For this review, take the finished solid that the model builds, in its own axes (mm). A direction names the side the tool comes from. Round coordinates to 2 decimals unless told otherwise and drop trailing zeros. Write each loop counter-clockwise with the first axis right and the second up, starting at its lowest first coordinate (ties: lowest second). Pieces come first, ordered by that corner, then holes. Notation, with made-up numbers: (64, 67.25) - (81, 67.25) arc R26 cw to (81, 97.25) - close; hole circle Ø9 at (20.25, 59.5). An arc over 180 degrees is marked (long way). One line per item, written item: value. Start each with the question number.
Q1. Mouldability with a two-part tool opening along Y and no side actions: class faces 3 (the face through (-0.524, 1.61, 1.663)), 4 (the face through (0, 6, 0)), 5 (the face through (-0.871, 3.481, 2.766)), 6 (the face through (-0.2, -0.3, 0.7)) as +Y half, -Y half, draft (parallel to the pull), parting line (faces both ways), or undercut.
Q2. Add section B-B on y = 4. Write out the cut boundary in (x, z).
Q3. Add section A-A on y = 0.25. Write out the cut boundary in (x, z).
Q4. Tool access review of faces 1 (the face through (0, -1.613, -2)), 2 (the face through (2.685, -0.599, -0.596)): name each direction out of +Z, -Z, +X, -X, +Y, -Y from which nothing blocks a thin tool from reaching the whole face with its end or side.
Q5. For probe 1 along Y at (x, z) = (0.15, -2.55); probe 2 along Y at (x, z) = (0.45, 2.35); probe 3 along X at (y, z) = (3, 0.1), list the stretches that pass through material, from the lowest coordinate up.
Q6. Clearance check with flat-ended pins moving along their axes: pin 1 Ø1 at (x, z) = (-1, 0) entering from -Y; pin 2 Ø1.1 at (x, z) = (0, 0) entering from -Y; pin 3 Ø2 at (x, y) = (-1, 2) entering from -Z. State where each tip first meets the part, or that it passes through.
```python
from build123d import *


with BuildPart() as part:
    # 스케치1 → 회전1 (revolve)
    with BuildSketch(Plane(origin=(0, 0, 0), x_dir=(0, 0, -1), z_dir=(1, 0, 0)), mode=Mode.PRIVATE) as revolve_1_sk:
        Polygon((0, 0), (0.495725515, 0), (1.75, -1.612980168), (2.75, -1.612980168), (2.75, 0.387019832), (1.743371525, 1.102989251), (1.743371525, 2.102989251), (2.9, 2.757946751), (2.9, 4.183903925), (1.356376494, 5.576732475), (0, 6), align=None)
    revolve(revolve_1_sk.sketch.rotate(Axis((0, 6, 0), (0, -1, 0)), 180), axis=Axis((0, 6, 0), (0, -1, 0)))


solid = part.part
```
Result set:
1. face 3: undercut
1. face 4: +Y half
1. face 5: draft
1. face 6: -Y half
2. outline: circle Ø5.8 at (0, 0)
3. outline: circle Ø5.5 at (0, 0)
4. face 1: +Z, -Z, +X, -X, -Y
4. face 2: -Y
5. probe 1: y = -1.61 to 0.53, 2.56 to 4.5
5. probe 2: y = -1.61 to 0.64, 2.47 to 4.64
5. probe 3: x = -2.9 to 2.9
6. pin 1: stops at y = -1.29
6. pin 2: stops at y = -0.07
6. pin 3: stops at z = -2.88
